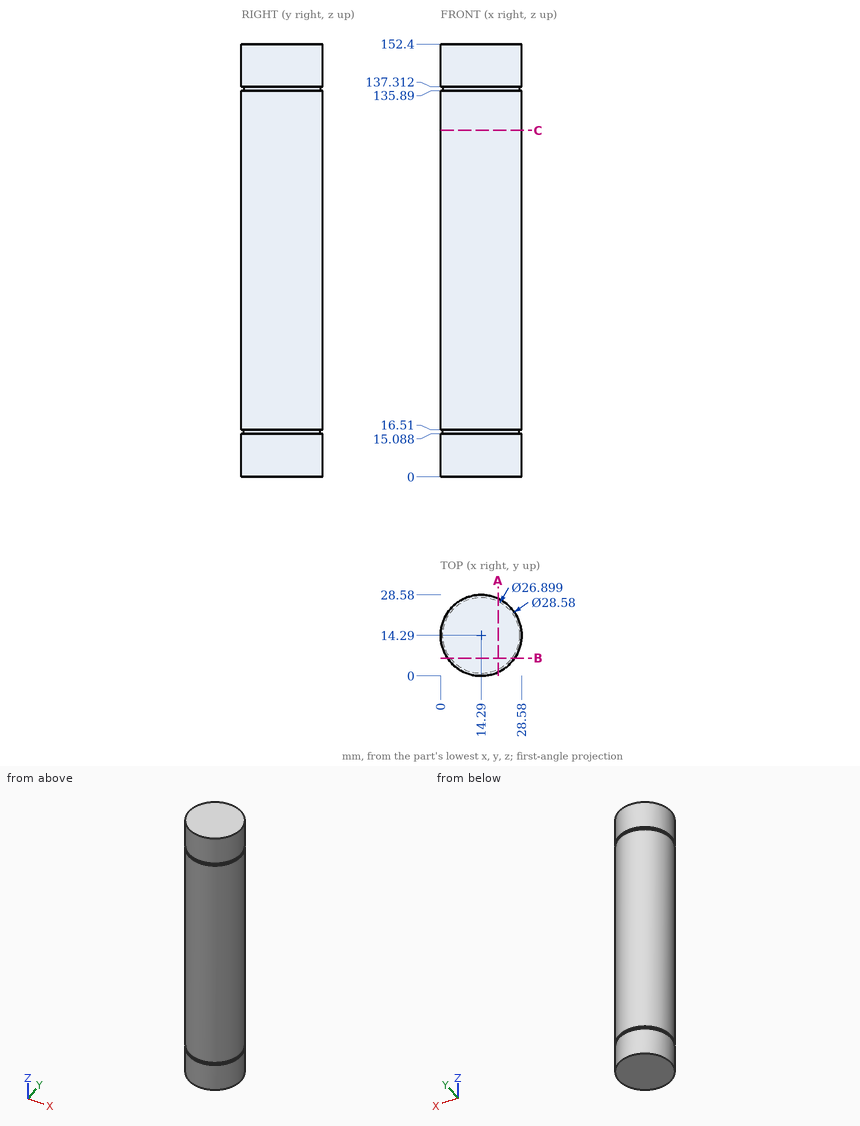
Source: three-view drawing plus pictorial views. Frame: mm from the lowest corner of the part. Round coordinates to 2 decimals unless told otherwise and drop trailing zeros. Loops run counter-clockwise (first coordinate to the right, second up) from the corner with the lowest first, then second, coordinate; pieces in that order, holes last.
Q1. Section B-B, the plane y = 6.25. Return loops of the section in (x, z).
Q2. Ray query, line 1 (Y direction, x = 15, z = 27.5); line 2 (X direction, y = 7.25, z = 24) (1 decimal); line 3 (Y direction, x = 24.25, z = 51) (1 decimal). Return the intervals inside material, ascending.
Q3. First-contact query: P1, Ø2, axis at y = 17, z = 80, coming from the +X side; P2, Ø3, axis at x = 10.5, z = 97, coming from the +Y side (1 decimal). Flat tips, straight axial feed; report the tip coordinate or a pass-through.
Q4. Section A-A, the plane x = 20.25. Return loops of the section in (y, z), plus the area to 3 significant figures.
Q5. Section C-C, the plane z = 122. Return loops of the section in (x, y).
Solutions:
1. outline: (2.48, 0) - (26.1, 0) - (26.1, 15.09) - (25.07, 15.09) - (25.07, 16.51) - (26.1, 16.51) - (26.1, 135.89) - (25.07, 135.89) - (25.07, 137.31) - (26.1, 137.31) - (26.1, 152.4) - (2.48, 152.4) - (2.48, 137.31) - (3.51, 137.31) - (3.51, 135.89) - (2.48, 135.89) - (2.48, 16.51) - (3.51, 16.51) - (3.51, 15.09) - (2.48, 15.09) - close
2. line 1: y = 0.02 to 28.56
2. line 2: x = 1.9 to 26.7
2. line 3: y = 4 to 24.5
3. P1: stops at x = 28.48
3. P2: stops at y = 28.4
4. outline: (1.3, 0) - (27.28, 0) - (27.28, 15.09) - (26.35, 15.09) - (26.35, 16.51) - (27.28, 16.51) - (27.28, 135.89) - (26.35, 135.89) - (26.35, 137.31) - (27.28, 137.31) - (27.28, 152.4) - (1.3, 152.4) - (1.3, 137.31) - (2.23, 137.31) - (2.23, 135.89) - (1.3, 135.89) - (1.3, 16.51) - (2.23, 16.51) - (2.23, 15.09) - (1.3, 15.09) - close
4. area: 3,950 mm2
5. outline: circle Ø28.58 at (14.29, 14.29)
